```python
from build123d import *

# Parameters (mm, degrees)
F0_W     = 127
F0_H     = 118
F1_DEPTH = 7
F2_R     = 1.1
F3_DEPTH = 25
F4_R     = 5.2
F5_DEPTH = 7.001
F6_R     = 5.2
F7_DEPTH = 7.001


with BuildPart() as f1:
    # F0 (on Top) → F1 (new body)
    with BuildSketch(Plane.XY):
        Rectangle(F0_W, F0_H)
    extrude(amount=F1_DEPTH)

    # F2 (on face) → F3 (cut)
    with BuildSketch(Plane(origin=(0, 0, 0), x_dir=(1, 0, 0), z_dir=(0, 0, -1))):
        with BuildLine():
            ThreePointArc((-55.5, -50.1), (-54.722183, -49.777817), (-54.4, -49))
            ThreePointArc((-54.4, -49), (-56.277817, -48.222183), (-55.5, -50.1))
        make_face()
        with Locations((55.5, -49)):
            Circle(F2_R)
        with Locations((-55.5, 49)):
            Circle(F2_R)
        with Locations((55.5, 49)):
            Circle(F2_R)
    extrude(amount=-F3_DEPTH, mode=Mode.SUBTRACT)

    # F4 (on Top) → F5 (cut, through all)
    with BuildSketch(Plane.XY):
        with Locations((-36, 30.4)):
            Circle(F4_R)
        with Locations((-36, -1.6)):
            Circle(F4_R)
        with Locations((0, -1.6)):
            Circle(F4_R)
        with Locations((34.7, -1.6)):
            Circle(F4_R)
        with Locations((34.7, 30.4)):
            Circle(F4_R)
        with Locations((0, 30.4)):
            Circle(F4_R)
    extrude(amount=F5_DEPTH, mode=Mode.SUBTRACT)

    # F6 (on face) → F7 (cut, through all)
    with BuildSketch(Plane.XY.offset(7)):
        with Locations((20.918876, -31.143876)):
            Circle(F6_R)
    extrude(amount=-F7_DEPTH, mode=Mode.SUBTRACT)


solid = f1.part
```
Can you work these out from the model? Positions are in its coordinate system, mm. Round coordinates to 2 decimals unless told otherwise and drop trailing zeros. Loops run counter-clockwise (first coordinate to the right, second up) from the corner with the lowest first, then second, coordinate; pieces in that order, holes last. Notation, with made-up numbers: (86, 20.5) -> (145, 20.5) arc R21 ccw to (145, 36.5) -> close; hole circle Ø8 at (63.25, -34). An arc over 180 degrees is marked (long way). One line per item, written item: value. Start each with the question number.
1. If we section it at C-C, the plane z = 3.25: Give the number of separate pieces and of enclosed holes in the cut face, then the cut area to 3 significant figures.
2. If we section it at D-D, the plane x = 1: Write out the boundary of the cut face in (y, z).
3. If we section it at B-B, the plane x = -36: Write out the boundary of the cut face in (y, z).
4. If I drill on probe 1 along Y at (x, z) = (0, 2.5); probe 2 along X at (y, z) = (30.4, 2.25); probe 3 along X at (y, z) = (-49, 4.75), over which ranges is the centre line in solid material (lowest first)?
5. If we section it at A-A, the plane y = 30.4: Write out the boundary of the cut face in (x, z), then the cut area to 3 significant figures.
6. If we mould it in two halves opening along X, with no side actions, what happens to faces 1 (the cylindrical face through (25.72, -33.14, 3.55)), 2 (the flat face through (-1, 59, 3)), 3 (the flat face through (-63.5, -1, 3))? For each: pulls with the +X half, pulls with the -X half, needs draft (parallel to the pull), parting line crosses it, or undercut.
Calculated:
1. separate pieces: 1
1. enclosed holes: 11
1. area: 14,400 mm²
2. outline: (-59, 0) -> (-6.7, 0) -> (-6.7, 7) -> (-59, 7) -> close; (3.5, 0) -> (25.3, 0) -> (25.3, 7) -> (3.5, 7) -> close; (35.5, 0) -> (59, 0) -> (59, 7) -> (35.5, 7) -> close
3. outline: (-59, 0) -> (-6.8, 0) -> (-6.8, 7) -> (-59, 7) -> close; (3.6, 0) -> (25.2, 0) -> (25.2, 7) -> (3.6, 7) -> close; (35.6, 0) -> (59, 0) -> (59, 7) -> (35.6, 7) -> close
4. probe 1: y = -59 to -6.8, 3.6 to 25.2, 35.6 to 59
4. probe 2: x = -63.5 to -41.2, -30.8 to -5.2, 5.2 to 29.5, 39.9 to 63.5
4. probe 3: x = -63.5 to -56.6, -54.4 to 54.4, 56.6 to 63.5
5. outline: (-63.5, 0) -> (-41.2, 0) -> (-41.2, 7) -> (-63.5, 7) -> close; (-30.8, 0) -> (-5.2, 0) -> (-5.2, 7) -> (-30.8, 7) -> close; (5.2, 0) -> (29.5, 0) -> (29.5, 7) -> (5.2, 7) -> close; (39.9, 0) -> (63.5, 0) -> (63.5, 7) -> (39.9, 7) -> close
5. area: 671 mm²
6. face 1: undercut
6. face 2: needs draft
6. face 3: pulls with the -X half
